Autodesk Inventor part; units mm, degrees
ref_plane "YZ Plane" through (0, 0, 0) normal (1, 0, 0) x (0, 1, 0)
ref_plane "XZ Plane" through (0, 0, 0) normal (0, 1, 0) x (-1, 0, 0)
ref_plane "XY Plane" through (0, 0, 0) normal (0, 0, 1) x (1, 0, 0)
sketch "Sketch1" plane through (0, 0, 0) normal (1, 0, 0) x (0, 1, 0)
  circle A0 centre (0, 0) radius 30
  dimension "d0" = 60
extrude "Extrusion1" add sketch "Sketch1" along normal blind 54
sketch "Sketch2" plane through (0, 0, 0) normal (0, 1, 0) x (-1, 0, 0)
  line L0 (-54, 30) -> (-54, -30)
  circle A0 centre (-54, 0) radius 47.5
  point P0 (0, 0)
  dimension "d3" = 95
extrude "Extrusion2" add sketch "Sketch2" along normal mid plane 60
move or copy body "Move Body1" bodies to move or copy 1 copy no translate (15, 0, 0)
properties part number "hip"
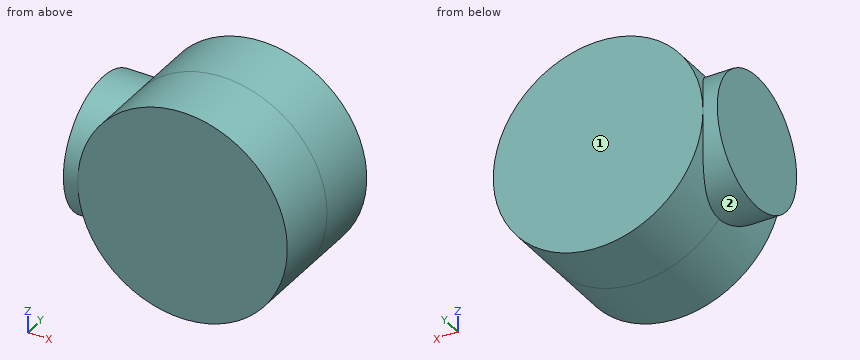
Read the model definition and answer for the solid it produces. Units are mm, in the model's axes. Face numbers are marked on the shaded views. A direction names the side the tool comes from. Round coordinates to 2 decimals unless told otherwise and drop trailing zeros. Write each loop counter-clockwise with the first axis right and the second up, starting at its lowest first coordinate (ties: lowest second). Pieces come first, ordered by that corner, then holes.
Q1. Find section D-D on z = -38.5. Determine the outline of the cut face in (x, y), and give its area (3 significant figures).
Values:
outline: (41.18, -30) - (96.82, -30) - (96.82, 30) - (41.18, 30) - close
area: 3,340 mm2
Q2. Find section A-A on z = -18. Determine the outline of the cut face in (x, y).
Values:
outline: (15, -24) - (25.04, -24) - (25.04, -30) - (112.96, -30) - (112.96, 30) - (25.04, 30) - (25.04, 24) - (15, 24) - close
Q3. Flat-ended cylindrical pins translate along their axes: P1, Ø1, axis at x = 57.5, y = -6, coming from the +Z side; P2, Ø8, axis at x = 26.5, y = 8.5, coming from the +Z side; P3, Ø8, axis at y = 18, z = 15, coming from the +X side. Find the tip coordinate at first contact, or state that the pin passes through.
Values:
P1: stops at z = 46.21
P2: stops at z = 29.66
P3: stops at x = 115.21
Q4. Straight lines are drawn through the part: line 1 (Z direction, x = 63, y = -13.5); line 2 (Z direction, x = 107.5, y = -20.5); line 3 (Y direction, x = 26, z = 21.5). For each, find the intervals that lie inside material, in ascending order.
Values:
line 1: z = -47.12 to 47.12
line 2: z = -27.82 to 27.82
line 3: y = -20.92 to 20.92
Q5. A tool of negligible diameter and unlimited length cuts with its end or side. For the marked faces 1 and 2, from which of +Z, -Z, +X, -X, +Y, -Y can it reach the whole face along a straight path? Write none if from no direction.
Values:
face 1: +Z, -Z, +X, -X, +Y
face 2: -X
Q6. Find section B-B on x = 30. Determine the outline of the cut face in (y, z).
Values:
outline: (-30, -27.12) - (-12.84, -27.12) arc R30 ccw to (12.84, -27.12) - (30, -27.12) - (30, 27.12) - (12.84, 27.12) arc R30 ccw to (-12.84, 27.12) - (-30, 27.12) - close
Q7. Find section C-C on y = -12. Determine the outline of the cut face in (x, z), and give its area (3 significant figures).
Values:
outline: (15, -27.5) - (30.27, -27.5) arc R47.5 ccw (long way) to (30.27, 27.5) - (15, 27.5) - close
area: 7,600 mm2
